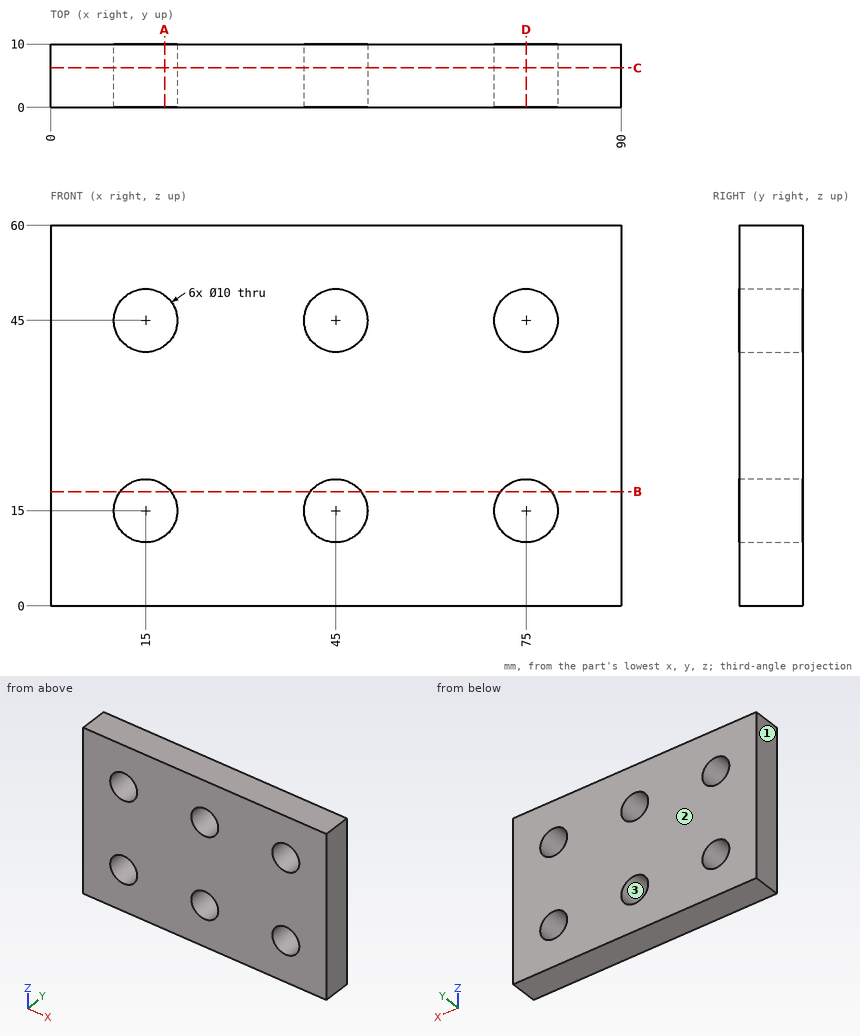
Geometry check sheet. Reference: drawing and pictorial views, mm from the part's lowest x, y, z. Round coordinates to 2 decimals unless told otherwise and drop trailing zeros. Order: outer loops, then holes, each group sorted by start corner. A loop starts at its lowest first (then second) coordinate and runs counter-clockwise, first axis right, second up.
Q1. Depth check by flat-ended pin: P1, Ø6, axis at x = 75, z = 15, coming from the +Y side. Enter the tip coordinate at first touch or a pass-through.
Filled sheet:
P1: passes through
Q2. Cross-section at D-D, the plane x = 75. Enter the section's corners in (y, z).
Filled sheet:
outline: (0, 0) - (10, 0) - (10, 10) - (0, 10) - close; (0, 20) - (10, 20) - (10, 40) - (0, 40) - close; (0, 50) - (10, 50) - (10, 60) - (0, 60) - close
Q3. Cross-section at B-B, the plane z = 18. Enter the section's corners in (x, y), plus the area to 3 significant figures.
Filled sheet:
outline: (0, 0) - (11, 0) - (11, 10) - (0, 10) - close; (19, 0) - (41, 0) - (41, 10) - (19, 10) - close; (49, 0) - (71, 0) - (71, 10) - (49, 10) - close; (79, 0) - (90, 0) - (90, 10) - (79, 10) - close
area: 660 mm2
Q4. Draft check along X on the marked faces 1, 2 and 3. Enter one of: pulls with the +X half, pulls with the -X half, needs draft (parallel to the pull), parting line crosses it, or undercut.
Filled sheet:
face 1: pulls with the -X half
face 2: needs draft
face 3: undercut
Q5. Scan lines: L1, parallel to Z at x = 15, y = 4.25; L2, parallel to X at y = 3, z = 15; L3, parallel to Z at x = 46.5, y = 5.5. Record each from-to range of solid material in increasing order.
Filled sheet:
L1: z = 0 to 10, 20 to 40, 50 to 60
L2: x = 0 to 10, 20 to 40, 50 to 70, 80 to 90
L3: z = 0 to 10.23, 19.77 to 40.23, 49.77 to 60
Q6. Cross-section at C-C, the plane y = 6.25. Enter the section's corners in (x, z).
Filled sheet:
outline: (0, 0) - (90, 0) - (90, 60) - (0, 60) - close; hole circle Ø10 at (15, 15); hole circle Ø10 at (15, 45); hole circle Ø10 at (45, 15); hole circle Ø10 at (45, 45); hole circle Ø10 at (75, 15); hole circle Ø10 at (75, 45)
Q7. Cross-section at A-A, the plane x = 18. Enter the section's corners in (y, z).
Filled sheet:
outline: (0, 0) - (10, 0) - (10, 11) - (0, 11) - close; (0, 19) - (10, 19) - (10, 41) - (0, 41) - close; (0, 49) - (10, 49) - (10, 60) - (0, 60) - close
